Build history of the part. All positions in model axes, mm. Face numbers are marked on the shaded views. A direction names the side the tool comes from. Give positions to 0.01 mm unless a question says otherwise; leave off trailing zeros. Write each loop counter-clockwise with the first axis right and the second up, starting at its lowest first coordinate (ties: lowest second). Pieces come first, ordered by that corner, then holes. Notation, with made-up numbers: (9.5, 0) -> (48.5, 0) arc R21 ccw to (48.5, 33) -> close; hole circle Ø6 at (-5.5, 70). An arc over 180 degrees is marked (long way). One line per question, with ' | ' between items. Start each with the question number.
(1) Band-saw the part on C-C, the plane y = 0. Give the cut face in (x, z), and give its area (3 significant figures).
(2) Band-saw the part on D-D, the plane z = 4.5. Give the cut face in (x, y).
(3) Band-saw the part on B-B, the plane x = 0. Give the cut face in (y, z).
(4) Drill centre lines: probe 1 along Y at (x, z) = (-0.25, 18.5); probe 2 along Z at (x, y) = (-7.5, -3.5); probe 3 along X at (y, z) = (-2.5, 4.75). Where is each one in solid material? Low to high. Write a range as from..to.
(5) Tool access for the marked faces 1, 2, 3 and 4: list every direction of +Z, -Z, +X, -X, +Y, -Y with a clear straight run to the whole face (end or side of a thin tool).
(6) Pin check, flat tips, straight feed: P1, Ø5, axis at y = 9, z = 4.5, coming from the -X side; P2, Ø2.5, axis at x = -6, y = -6.5, coming from the +Z side; P3, Ø3, axis at y = -8, z = 16, coming from the +X side. Stop position of each tip, or through.
(7) Band-saw the part on A-A, the plane z = 10.25. Give the cut face in (x, y).
(8) Pull direction Z, two halves, no side cores. Call the marked faces 5, 6, 7 and 8: released by +Z, released by -Z, zero draft, split by the parting line, or undercut.
from build123d import *

# Parameters (mm, degrees)
ESBO_O1_R                 = 12.5
RESSALTO_EXTRUS_O1_DEPTH  = 20
CORTE_EXTRUS_O3_DEPTH     = 11
ESBO_O3_R                 = 4
CORTE_EXTRUS_O4_DEPTH     = 21
ESBO_O6_W                 = 12
ESBO_O6_H                 = 2
CORTE_EXTRUS_O5_DEPTH     = 10
CORTE_EXTRUS_O6_START     = -3
ESBO_O7_R                 = 3.25
CORTE_EXTRUS_O6_DEPTH     = 9.5
FURO_ROSCADO_DE_M3X0_51_D = 2.5
FILETE1_R                 = 1
ESBO_O10_R                = 1.5
CORTE_EXTRUS_O7_DEPTH     = 1
CHANFRO1_SIZE             = 0.5
CORTE_EXTRUS_O8_REACH     = 18.5
ESBO_O11_R                = 1.5
ESBO_O12_R                = 6
CORTE_EXTRUS_O9_DEPTH     = 11
PADR_OCIRCULAR1_COUNT     = 4
CHANFRO2_SIZE             = 0.5


with BuildPart() as part:
    # Esboço1 → Ressalto-extrusão1 (new body)
    with BuildSketch(Plane.XY):
        Circle(ESBO_O1_R)
    extrude(amount=RESSALTO_EXTRUS_O1_DEPTH)

    # Esboço2 → Corte-extrusão3 (cut)
    with BuildSketch(Plane.XY.offset(20)):
        with BuildLine():
            Line((0, 0), (6.25, 10.825317547))
            ThreePointArc((6.25, 10.825317547), (12.5, 0), (6.25, -10.825317547))
            Line((6.25, -10.825317547), (0, 0))
        make_face()
    corte_extrus_o3 = extrude(amount=-CORTE_EXTRUS_O3_DEPTH, mode=Mode.SUBTRACT)

    # Esboço3 → Corte-extrusão4 (cut, through all)
    with BuildSketch(Plane(origin=(0, 0, 0), x_dir=(-1, 0, 0), z_dir=(0, 0, -1))):
        Circle(ESBO_O3_R)
    extrude(amount=-CORTE_EXTRUS_O4_DEPTH, mode=Mode.SUBTRACT)

    # Espelhar1: Corte-extrusão3 across plane
    add(corte_extrus_o3.mirror(Plane(origin=(0, 0, 0), x_dir=(0, 0, 1), z_dir=(1, 0, 0))), mode=Mode.SUBTRACT)

    # Esboço6 → Corte-extrusão5 (cut, through all)
    with BuildSketch(Plane.XY.offset(9)):
        with Locations((7, 0)):
            Rectangle(ESBO_O6_W, ESBO_O6_H)
    extrude(amount=-CORTE_EXTRUS_O5_DEPTH, mode=Mode.SUBTRACT)

    # Esboço7 → Corte-extrusão6 (cut, through all)
    with BuildSketch(Plane.XZ.offset(-1).offset(CORTE_EXTRUS_O6_START)):
        with Locations((8.459935794, 4.5)):
            Circle(ESBO_O7_R)
    extrude(amount=-CORTE_EXTRUS_O6_DEPTH, mode=Mode.SUBTRACT)

    # Furo roscado de M3x0.51 (through all)
    with Locations(Plane(origin=(0, 4, 0), x_dir=(1, 0, 0), z_dir=(0, 1, 0))):
        with Locations((8.459935794, -4.5)):
            Hole(FURO_ROSCADO_DE_M3X0_51_D / 2)

    # Filete1
    filete1_edges = [part.edges().sort_by_distance(p)[0] for p in [
        (-12.5, 0, 0),
    ]]
    fillet(filete1_edges, radius=FILETE1_R)

    # Esboço10 → Corte-extrusão7 (cut)
    with BuildSketch(Plane.XY.offset(9)):
        with Locations((6.363961031, -6.363961031)):
            Circle(ESBO_O10_R)
    corte_extrus_o7 = extrude(amount=-CORTE_EXTRUS_O7_DEPTH, mode=Mode.SUBTRACT)

    # Chanfro1
    chanfro1_edges = [part.edges().sort_by_distance(p)[0] for p in [
        (0, -12.5, 20),
        (0, 12.5, 20),
    ]]
    chamfer(chanfro1_edges, length=CHANFRO1_SIZE)

    # Esboço11 → Corte-extrusão8 (cut, up to next)
    with BuildSketch(Plane(origin=(0, 4, 0), x_dir=(1, 0, 0), z_dir=(0, 1, 0)), mode=Mode.PRIVATE) as corte_extrus_o8_sk1:
        with Locations((8.459935794, -4.5)):
            Circle(ESBO_O11_R)
    corte_extrus_o8_tool1 = extrude(corte_extrus_o8_sk1.sketch, amount=-CORTE_EXTRUS_O8_REACH, mode=Mode.PRIVATE) & part.part
    add(corte_extrus_o8_tool1.solids().sort_by_distance((8.459936, 4, 4.5))[0], mode=Mode.SUBTRACT)

    # Esboço12 → Corte-extrusão9 (cut)
    with BuildSketch(Plane.XY.offset(20)):
        Circle(ESBO_O12_R)
    extrude(amount=-CORTE_EXTRUS_O9_DEPTH, mode=Mode.SUBTRACT)

    # PadrãoCircular1: Corte-extrusão7 ×4 about axis
    padr_ocircular1_axis = Axis((0, 0, 0), (0, 0, 1))
    for i in range(1, PADR_OCIRCULAR1_COUNT):
        add(corte_extrus_o7.rotate(padr_ocircular1_axis, i * 360 / PADR_OCIRCULAR1_COUNT), mode=Mode.SUBTRACT)

    # Chanfro2
    chanfro2_edges = [part.edges().sort_by_distance(p)[0] for p in [
        (-4, 0, 0),
    ]]
    chamfer(chanfro2_edges, length=CHANFRO2_SIZE)


solid = part.part
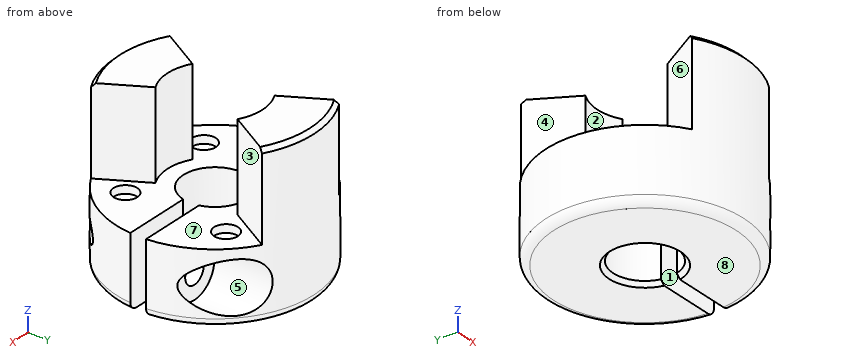
Results:
1) outline: (-12.5, 1) arc R1 ccw to (-11.5, 0) -> (-4.5, 0) -> (-4, 0.5) -> (-4, 9) -> (-12.5, 9) -> close | area: 76.2 mm²
2) outline: (3.87, -1) arc R4 cw (long way) to (3.87, 1) -> (6.96, 1) -> (6.96, 4) -> (5.21, 4) -> (5.21, 11.36) arc R12.5 ccw (long way) to (7.21, -10.21) -> (7.21, -1) -> close; (9.71, -7.87) arc R12.5 ccw to (12.46, -1) -> (9.71, -1) -> close; (9.96, 1) -> (12.46, 1) arc R12.5 ccw to (11.71, 4.37) -> (11.71, 4) -> (9.96, 4) -> close
3) outline: (-12.5, 1) arc R1 ccw to (-11.5, 0) -> (-4.5, 0) -> (-4, 0.5) -> (-4, 9) -> (-6, 9) -> (-6, 20) -> (-12, 20) -> (-12.5, 19.5) -> close; (4, 0.5) -> (4.5, 0) -> (11.5, 0) arc R1 ccw to (12.5, 1) -> (12.5, 19.5) -> (12, 20) -> (6, 20) -> (6, 9) -> (4, 9) -> close
4) probe 1: y = -12.5..-5.99, 5.99..12.5 | probe 2: z = 0..9 | probe 3: x = -12.25..-3.12, 3.12..7.24, 9.68..12.25
5) face 1: +Z, -Z, +X | face 2: +Z | face 3: +Z, +X | face 4: +Z, -X
6) P1: stops at x = -10.68 | P2: stops at z = 9 | P3: stops at x = 5.48
7) outline: (-6.25, -10.83) arc R12.5 ccw to (6.25, -10.83) -> (3, -5.2) arc R6 cw to (-3, -5.2) -> close; (-6.25, 10.83) -> (-3, 5.2) arc R6 cw to (3, 5.2) -> (6.25, 10.83) arc R12.5 ccw to start
8) face 5: undercut | face 6: zero draft | face 7: released by +Z | face 8: released by -Z
